Verification items for this drawing (mm, ordinates from the low corner). A direction names the side the tool comes from. Round coordinates to 2 decimals unless told otherwise and drop trailing zeros. Order: outer loops, then holes, each group sorted by start corner. A loop starts at its lowest first (then second) coordinate and runs counter-clockwise, first axis right, second up. Notation, with made-up numbers: M 36,-39.5 L 77,-39.5 A11 cw 77,-32.5 Z; hole C 43.5,-2.75 d3. An arc over 180 degrees is marked long. One line per item, written item: value. Start each with the question number.
(1) Access from +Z, -Z, +X, -X, +Y, -Y to the whole of each face (thin tool, end or side, straight path). Record for the marked faces 4 and 5.
(2) Cross-section at D-D, the plane z = 24. Enter the section's corners in (x, y).
(3) Cross-section at A-A, the plane x = 13.25. Enter the section's corners in (y, z).
(4) Thickness scan on L1, parallel to Y at x = 13.25, z = 45.35; L2, parallel to Z at x = 15.75, y = 16.5; L3, parallel to Y at x = 13.5, z = 25. Record the ranges inside material, lowest first.
(5) Cross-section at C-C, the plane z = 44.5. Enter the section's corners in (x, y).
(6) Release check for a two-part mould opening along Y. For the marked faces 1, 2 and 3 record: released by +Y, released by -Y, zero draft, split by the parting line, or undercut.
(7) Depth check by flat-ended pin: pin 1 Ø1 at (y, z) = (3.5, 5) entering from +X; pin 2 Ø5 at (x, z) = (10, 8) entering from +Y; pin 3 Ø5 at (x, z) = (16, 37) entering from -Y. Enter the tip coordinate at first touch or a pass-through.
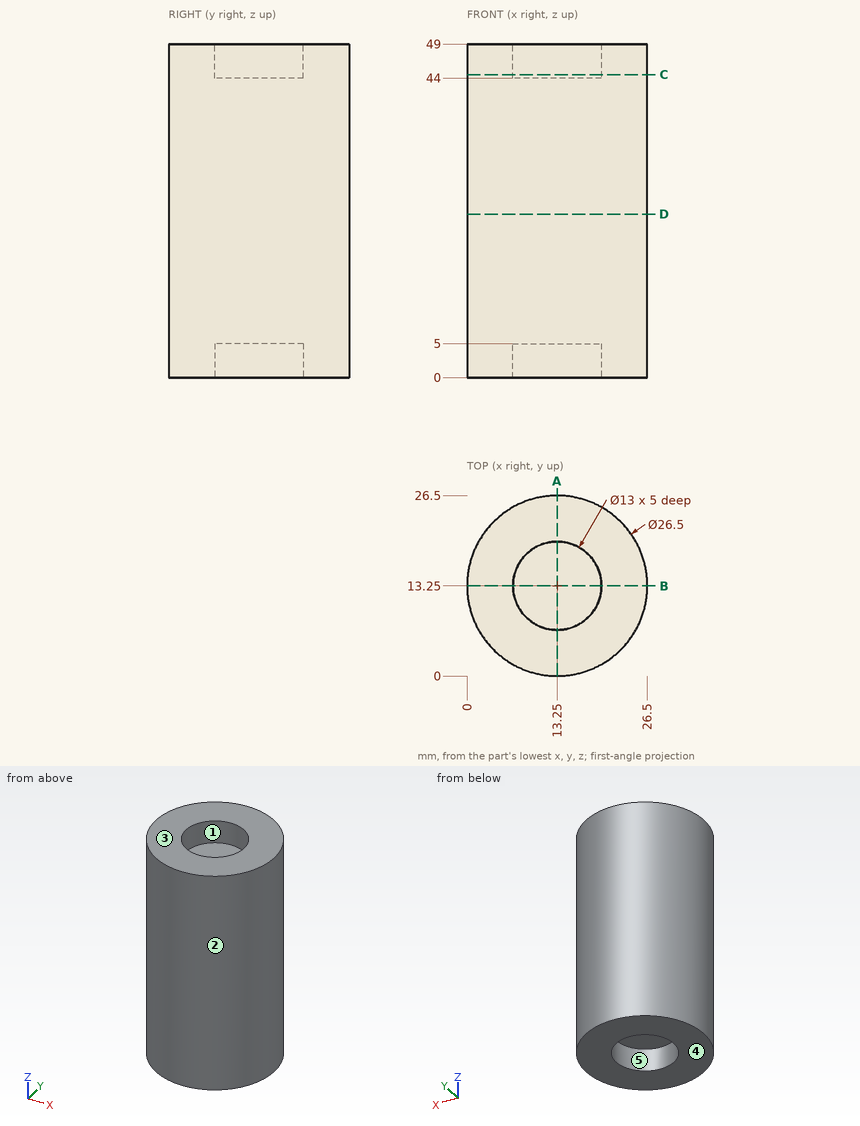
Values found:
1. face 4: -Z, +X, -X, +Y, -Y
1. face 5: -Z
2. outline: C 13.25,13.25 d26.5
3. outline: M 0,0 L 6.75,0 L 6.75,5 L 19.75,5 L 19.75,0 L 26.5,0 L 26.5,49 L 19.75,49 L 19.75,44 L 6.75,44 L 6.75,49 L 0,49 Z
4. L1: 0 to 6.75, 19.75 to 26.5
4. L2: 5 to 44
4. L3: 0 to 26.5
5. outline: C 13.25,13.25 d26.5; hole C 13.25,13.25 d13
6. face 1: undercut
6. face 2: split by the parting line
6. face 3: zero draft
7. pin 1: x = 22.74
7. pin 2: y = 26.48
7. pin 3: y = 0
